from build123d import *

# Parameters (mm, degrees)
SKETCH1_R           = 7.5
SKETCH1_R_2         = 1.6
BOSS_EXTRUDE1_DEPTH = 2


with BuildPart() as part:
    # Sketch1 → Boss-Extrude1 (new body)
    with BuildSketch(Plane(origin=(0, 0, 0), x_dir=(1, 0, 0), z_dir=(0, 1, 0))):
        with Locations(Location((0, 0, 0), (0, 0, 270))):
            Circle(SKETCH1_R)
        with Locations(Location((0, 0, 0), (0, 0, 270))):
            Circle(SKETCH1_R_2, mode=Mode.SUBTRACT)
        with BuildLine():
            Line((-1.319908308, 3.186540538), (-2.104758878, 5.081337429))
            ThreePointArc((-2.104758878, 5.081337429), (-3.889087297, 3.889087297), (-5.081337429, 2.104758878))
            Line((-5.081337429, 2.104758878), (-3.186540538, 1.319908308))
            ThreePointArc((-3.186540538, 1.319908308), (-2.438872541, 2.438872541), (-1.319908308, 3.186540538))
        make_face(mode=Mode.SUBTRACT)
        with BuildLine():
            Line((1.319908308, 3.186540538), (2.104758878, 5.081337429))
            ThreePointArc((2.104758878, 5.081337429), (3.889087297, 3.889087297), (5.081337429, 2.104758878))
            Line((5.081337429, 2.104758878), (3.186540538, 1.319908308))
            ThreePointArc((3.186540538, 1.319908308), (2.438872541, 2.438872541), (1.319908308, 3.186540538))
        make_face(mode=Mode.SUBTRACT)
        with BuildLine():
            Line((3.186540538, -1.319908308), (5.081337429, -2.104758878))
            ThreePointArc((5.081337429, -2.104758878), (3.889087297, -3.889087297), (2.104758878, -5.081337429))
            Line((2.104758878, -5.081337429), (1.319908308, -3.186540538))
            ThreePointArc((1.319908308, -3.186540538), (2.438872541, -2.438872541), (3.186540538, -1.319908308))
        make_face(mode=Mode.SUBTRACT)
        with BuildLine():
            Line((-1.319908308, -3.186540538), (-2.104758878, -5.081337429))
            ThreePointArc((-2.104758878, -5.081337429), (-3.889087297, -3.889087297), (-5.081337429, -2.104758878))
            Line((-5.081337429, -2.104758878), (-3.186540538, -1.319908308))
            ThreePointArc((-3.186540538, -1.319908308), (-2.438872541, -2.438872541), (-1.319908308, -3.186540538))
        make_face(mode=Mode.SUBTRACT)
    extrude(amount=BOSS_EXTRUDE1_DEPTH)


solid = part.part
Here's how the part is built. I have some questions about the finished solid (model axes, mm). A direction names the side the tool comes from. Coordinates: 2 decimals unless noted, no trailing zeros. Order: outer loops, then holes, each group sorted by start corner. A loop starts at its lowest first (then second) coordinate and runs counter-clockwise, first axis right, second up. Notation, with made-up numbers: (-26.5, 21.5) -> (-22.5, 21.5) arc R11 ccw to (-22.5, 28.5) -> close; hole circle Ø1 at (35, 62.25). An arc over 180 degrees is marked (long way). Answer in a Markdown table with one row per item.
(1) Please list where these lines run through material, in increasing order: probe 1 along X at (y, z) = (1.5, 0); probe 2 along X at (y, z) = (1.05, 3); probe 3 along X at (y, z) = (1, 3.25).
Answer key:
| item | result |
|---|---|
| probe 1 | -7.5 to -1.6, 1.6 to 7.5 |
| probe 2 | -6.87 to -4.61, -1.7 to 1.7, 4.61 to 6.87 |
| probe 3 | -6.76 to -4.44, -1.35 to 1.35, 4.44 to 6.76 |
(2) Thinking about a two-plate mould opening in Z: for faces 3 (the face through (2, 0, 0)), 4 (the face through (-3.87, 0.99, 3.91)), 5 (the face through (0.33, 0.986, -7.493)), which applies, +Z half, -Z half, draft (parallel to the pull), parting line (faces both ways), or undercut?
Answer key:
| item | result |
|---|---|
| face 3 | draft |
| face 4 | undercut |
| face 5 | parting line |
(3) Will this pin go through, and if not, where does the flat tip stop? pin 1 Ø1 at (x, y) = (-3, 1.5) entering from +Z.
Answer key:
| item | result |
|---|---|
| pin 1 | z = 7.07 |
(4) I want a section at B-B on z = 0. List the corners of the cut face in (x, y) for me, then the cut area to 3 significant figures.
Answer key:
| item | result |
|---|---|
| outline | (-7.5, 0) -> (-1.6, 0) -> (-1.6, 2) -> (-7.5, 2) -> close; (1.6, 0) -> (7.5, 0) -> (7.5, 2) -> (1.6, 2) -> close |
| area | 23.6 mm^2 |
(5) I want a section at C-C on y = 1.55. List the corners of the cut face in (x, z) for me.
Answer key:
| item | result |
|---|---|
| outline | circle Ø15 at (0, 0); hole (-5.08, -2.1) arc R5.5 ccw to (-2.1, -5.08) -> (-1.32, -3.19) arc R3.45 cw to (-3.19, -1.32) -> close; hole (-5.08, 2.1) -> (-3.19, 1.32) arc R3.45 cw to (-1.32, 3.19) -> (-2.1, 5.08) arc R5.5 ccw to start; hole circle Ø3.2 at (0, 0); hole (1.32, -3.19) -> (2.1, -5.08) arc R5.5 ccw to (5.08, -2.1) -> (3.19, -1.32) arc R3.45 cw to start; hole (1.32, 3.19) arc R3.45 cw to (3.19, 1.32) -> (5.08, 2.1) arc R5.5 ccw to (2.1, 5.08) -> close |
(6) I want a section at A-A on x = 0. List the corners of the cut face in (y, z) for me.
Answer key:
| item | result |
|---|---|
| outline | (0, -7.5) -> (2, -7.5) -> (2, -1.6) -> (0, -1.6) -> close; (0, 1.6) -> (2, 1.6) -> (2, 7.5) -> (0, 7.5) -> close |
(7) On a 3-axis mill with a long thin cutter (end or side, diameter ignored), from which of +Z, -Z, +X, -X, +Y, -Y can I reach the whole of each face in a straight line? I mean faces 1 (the face through (-4.1, 1, 1.7)), 2 (the face through (2, 2, 0)). Say none if no direction works.
Answer key:
| item | result |
|---|---|
| face 1 | +Y, -Y |
| face 2 | +Z, -Z, +X, -X, +Y |
(8) I want a section at D-D on x = -3. List the corners of the cut face in (y, z) for me, then the cut area to 3 significant figures.
Answer key:
| item | result |
|---|---|
| outline | (0, -6.87) -> (2, -6.87) -> (2, -4.61) -> (0, -4.61) -> close; (0, -1.7) -> (2, -1.7) -> (2, 1.7) -> (0, 1.7) -> close; (0, 4.61) -> (2, 4.61) -> (2, 6.87) -> (0, 6.87) -> close |
| area | 15.9 mm^2 |
